Verification items for the finished model (mm, model axes). Round coordinates to 2 decimals unless told otherwise and drop trailing zeros. Write each loop counter-clockwise with the first axis right and the second up, starting at its lowest first coordinate (ties: lowest second). Pieces come first, ordered by that corner, then holes. Notation, with made-up numbers: (36.5, -4.75) -> (45.5, -4.75) arc R10 ccw to (45.5, 0.25) -> close; hole circle Ø4 at (29, 28.25). An arc over 180 degrees is marked (long way). Answer as a JSON object with one key per item and string values. Group by question number.
(1) Sectioned sample at A-A on y = 12.5. Record the cut outline in (x, z).
(2) Sectioned sample at D-D on x = -47. Record the cut outline in (y, z).
(3) Sectioned sample at B-B on z = 22.15. Record the cut outline in (x, y).
(4) Scan lines: L1, parallel to Y at x = -52.5, z = 21.9; L2, parallel to X at y = 11.75, z = 20.6; L3, parallel to Y at x = -126, z = 23.5. Record each from-to range of solid material in increasing order. Write a range as from..to.
(5) Draft check along X on faces 1 (the face through (-129.498, 12.588, 22.042)), 2 (the face through (-52.76, 14.483, 22.042)), 3 (the face through (-40.003, 12.225, 22.042)), 4 (the face through (-89, 12, 19)). Enter one of: released by +X, released by -X, zero draft, split by the parting line, or undercut.
(6) Gauge pin test, flat end, axial feed: pin 1 Ø1.5 at (y, z) = (15.5, 23) entering from +X. Record the tip position at first contact, or that the pin passes through.
(7) Sectioned sample at C-C on y = 6.75. Record the cut outline in (x, z).
Autodesk Inventor part; units mm, degrees
ref_plane "YZ Plane" through (0, 0, 0) normal (1, 0, 0) x (0, 1, 0)
ref_plane "XZ Plane" through (0, 0, 0) normal (0, 1, 0) x (-1, 0, 0)
ref_plane "XY Plane" through (0, 0, 0) normal (0, 0, 1) x (1, 0, 0)
sketch "Sketch1" plane through (0, 0, 0) normal (0, 0, 1) x (1, 0, 0)
  line L0 (0, 0) -> (-140, 0)
  line L1 (-140, 0) -> (-140, 25)
  line L2 (-140, 25) -> (0, 25)
  line L3 (0, 25) -> (0, 0)
  dimension "d0" = 140
  dimension "d1" = 25
extrude "Extrusion1" add sketch "Sketch1" along normal blind 25
sketch "Sketch4" plane through (0, 0, 25) normal (0, 0, 1) x (1, 0, 0)
  point P0 (0, 0)
sketch "Sketch5" plane through (0, 0, 25) normal (0, 0, 1) x (1, 0, 0)
  line L0 (0, 25) -> (-140, 25)
  line L1 (0, 0) -> (-40, 0)
  line L2 (-40, 0) -> (-40, 25)
  line L3 (-40, 25) -> (0, 25)
  line L4 (0, 25) -> (0, 0)
  dimension "d16" = 40
extrude "Extrusion4" cut sketch "Sketch5" against normal blind 100
sketch "Sketch6" plane through (-40, 0, 25) normal (1, 0, 0) x (0, 0, -1)
  line L0 (25, 25) -> (0, 25)
  line L1 (25, 0) -> (6, 0)
  line L2 (6, 0) -> (6, 25)
  line L3 (6, 25) -> (25, 25)
  line L4 (25, 25) -> (25, 0)
  dimension "d19" = 19
extrude "Extrusion5" cut sketch "Sketch6" against normal blind 100
sketch "Sketch7" plane through (0, 0, 25) normal (0, 0, 1) x (1, 0, 0)
  circle A0 centre (-52.5, 12.5) radius 12.5
  circle A1 centre (-127.5, 12.5) radius 12.5
  line L0 (-40, 0) -> (-40, 25)
  line L1 (-140, 0) -> (-40, 0)
  line L2 (-140, 25) -> (-140, 0)
  circle A2 centre (-127.5, 12.5) radius 2
  circle A3 centre (-52.5, 12.5) radius 2
  line L3 (-40, 25) -> (-140, 25)
  point P0 (0, 0)
  point P1 (-52.5, 25)
  point P2 (-40, 12.5)
  point P3 (-52.5, 0)
  point P4 (-127.5, 25)
  point P5 (-140, 12.5)
  point P6 (-127.5, 0)
  dimension "d22" = 25
  dimension "d23" = 25
  dimension "d24" = 12.5
  dimension "d25" = 12.5
  dimension "d26" = 12.5
  dimension "d27" = 12.5
  dimension "d28" = 4
  dimension "d29" = 4
extrude "Extrusion6" cut sketch "Sketch7" against normal blind 100 contours L0 L1 A0 | A0 L3 L0 | A1 L2 L3 | L1 L2 A1 | A2 | A3
properties part number "Large Rod"
Computed values:
{
 "1": {"outline": "(-140, 19) -> (-129.5, 19) -> (-129.5, 25) -> (-140, 25) -> close; (-125.5, 19) -> (-54.5, 19) -> (-54.5, 25) -> (-125.5, 25) -> close; (-50.5, 19) -> (-40, 19) -> (-40, 25) -> (-50.5, 25) -> close"},
 "2": {"outline": "(1.28, 19) -> (23.72, 19) -> (23.72, 25) -> (1.28, 25) -> close"},
 "3": {"outline": "(-127.5, 0) -> (-52.5, 0) arc R12.5 ccw to (-52.5, 25) -> (-127.5, 25) arc R12.5 ccw to start; hole circle Ø4 at (-127.5, 12.5); hole circle Ø4 at (-52.5, 12.5)"},
 "4": {"L1": "0..10.5, 14.5..25", "L2": "-139.98..-129.35, -125.65..-54.35, -50.65..-40.02", "L3": "0..11.18, 13.82..25"},
 "5": {"face 1": "undercut", "face 2": "undercut", "face 3": "released by +X", "face 4": "zero draft"},
 "6": {"pin 1": "x = -40.2"},
 "7": {"outline": "(-138.6, 19) -> (-41.4, 19) -> (-41.4, 25) -> (-138.6, 25) -> close"}
}
